The model under review builds one solid part; all positions refer to its coordinate system, in mm. Face numbers are marked on the shaded views. A direction names the side the tool comes from. Give positions to 0.01 mm unless a question says otherwise; leave off trailing zeros. Order: outer loops, then holes, each group sorted by start corner. A loop starts at its lowest first (then second) coordinate and runs counter-clockwise, first axis right, second up. Notation, with made-up numbers: (87.25, -36.5) - (94.25, -36.5) arc R19 ccw to (94.25, 0.5) - close; hole circle Ø8 at (-25, 4.5). An arc over 180 degrees is marked (long way). Answer as CSV lines item,"result". Start each with the question number.
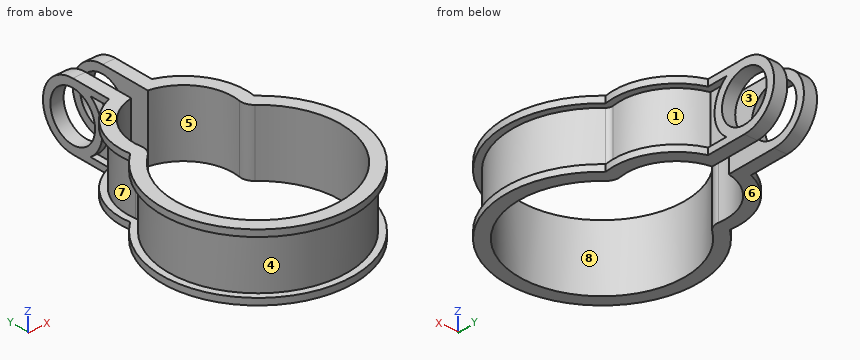
Autodesk Inventor part; units mm, degrees
ref_plane "Work Plane1" through (-2.5, 39.7902, 10) normal (1, 0, 0) x (0, 1, 0)
ref_plane "XZ Plane" through (0, 0, 0) normal (0, 1, 0) x (-1, 0, 0)
ref_plane "XY Plane" through (0, 0, 0) normal (0, 0, 1) x (1, 0, 0)
sketch "Sketch1" plane through (0, 0, 0) normal (0, 0, 1) x (1, 0, 0)
  arc A0 (-16.1874, 19.0517) -> (16.1874, 19.0517) centre (0, 0) ccw
  line L0 (-2.5, 50.7018) -> (-2.5, 39.7902) construction
  line L1 (2.5, 50.7018) -> (2.5, 39.7902) construction
  line L2 (2.5, 50.7018) -> (-2.5, 50.7018) construction
  arc A1 (14.8242, 22.7105) -> (2.5, 39.7902) centre (0, 25) ccw
  arc A2 (-2.5, 39.7902) -> (-14.8242, 22.7105) centre (0, 25) ccw
  arc A3 (-16.1874, 19.0517) -> (-14.8242, 22.7105) centre (-18.7774, 22.1) ccw
  arc A4 (14.8242, 22.7105) -> (16.1874, 19.0517) centre (18.7774, 22.1) ccw
  dimension "d0" = 25
  dimension "d2" = 25
  dimension "d3" = 5
  dimension "d4" = 4
sketch "Sketch2" plane through (0, 0, 0) normal (1, 0, 0) x (0, 1, 0)
  line L0 (-25, 10) -> (-25, -10)
  line L1 (-25, -10) -> (-29, -10)
  line L2 (-29, -10) -> (-29, -8)
  line L3 (-29, -8) -> (-27, -8)
  line L4 (-27, -8) -> (-27, 8)
  line L5 (-27, 8) -> (-29, 8)
  line L6 (-29, 8) -> (-29, 10)
  line L7 (-29, 10) -> (-25, 10)
  line L8 (19.0517, 0) -> (-25, 0)
  point P0 (0, 0)
  point P1 (19.0517, 0)
  dimension "d5" = 20
  dimension "d6" = 2
  dimension "d8" = 4
  dimension "d9" = 2
sweep "Sweep1" add profiles "Sketch2" path "Sketch1"
ref_plane "Work Plane1" through (-2.5, 39.7902, 10) normal (1, 0, 0) x (0, 1, 0)
sketch "Sketch3" plane through (-2.5, 39.7902, 10) normal (1, 0, 0) x (0, 1, 0)
  line L0 (0, 0) -> (0, -20)
  line L1 (0, -20) -> (15.2098, -20)
  arc A0 (15.2098, -20) -> (15.2098, 0) centre (15.2098, -10) ccw
  line L2 (15.2098, 0) -> (0, 0)
  line L3 (3.9441, 0) -> (3.9441, -2)
  point P0 (-39.7902, -10)
  dimension "d12" = 55
extrude "Extrusion1" add sketch "Sketch3" against normal blind 2
sketch "Sketch4" plane through (-4.5, 39.7902, 10) normal (-1, 0, 0) x (0, 0, 1)
  line L0 (-2, 3.6692) -> (-2, 1.6034) construction
  line L1 (0, 3.6692) -> (0, 15.2098)
  arc A0 (0, 15.2098) -> (-20, 15.2098) centre (-10, 15.2098) ccw
  line L2 (-20, 15.2098) -> (-20, 3.6692)
  arc A1 (-18, 9.2098) -> (-2, 9.2098) centre (-10, 15.2098) ccw
  line L3 (-20, 3.6692) -> (-20, 1.6034)
  line L4 (-20, 3.9441) -> (-20, 0)
  line L5 (-18, 1.6034) -> (-18, 9.2098)
  line L6 (-18, 1.972) -> (-18, 3.9441)
  line L7 (-18, 1.6034) -> (-20, 1.6034)
  line L8 (0, 3.6692) -> (0, 1.6034)
  line L9 (0, -17.6902) -> (0, 3.9441)
  line L10 (0, 1.6034) -> (-2, 1.6034)
  line L11 (-2, 1.6034) -> (-2, 9.2098)
  point P0 (-10, -39.7902)
extrude "Extrusion2" add sketch "Sketch4" along normal blind 2
mirror "Mirror1" about plane through (0, 0, 0) normal (1, 0, 0) of "Extrusion1", "Extrusion2"
sketch "Sketch5" plane through (-6.5, 39.7902, 10) normal (-1, 0, 0) x (0, 0, 1)
  arc A0 (0, 15.2098) -> (-20, 15.2098) centre (-10, 15.2098) ccw
  point P0 (-10, -39.7902)
hole "Hole1" at (-6.5, 55, 0) direction (1, 0, 0) diameter 15 end through all
properties part number "Part015. Double clip" material "Steel, Carbon"
Item 1: Take a section at A-A on y = 0. Write out the cut boundary in (x, z), and give its area (3 significant figures).
Item 2: For line 1 along X through (y, z) = (0, 3.75); line 2 along Z through (x, y) = (5, 55); line 3 along X through (y, z) = (25, 3.75), list the stretches that pass through material, from the lowest coordinate up.
Item 3: Take a section at C-C on x = 0. Write out the cut boundary in (y, z).
Item 4: Take a section at D-D on x = -21. Write out the cut boundary in (y, z).
Item 5: Clearance check with flat-ended pins moving along their axes: pin 1 (1.5 mm diameter, centred on y = 30, z = -2.5, fed in from -X); pin 2 (1 mm diameter, centred on x = -11, z = 0.5, fed in from -Y); pin 3 (2 mm diameter, centred on y = 37.5, z = -6, fed in from +X); pin 4 (9 mm diameter, centred on y = 55, z = 0, fed in from +X). State where each tip first meets the part, or that it passes through.
Item 6: Mouldability with a two-part tool opening along Z and no side actions: class the marked faces 6, 7 and 8 as released by +Z, released by -Z, zero draft, split by the parting line, or undercut.
Item 7: Machinability: for the marked faces 1, 2, 3, 4 and 5, which of the approach directions +Z, -Z, +X, -X, +Y, -Y give a long, thin tool a straight path to every point of the face, cutting with its end or side? Answer none if there is none.
Item 8: Take a section at B-B on z = 2. Count the separate pieces of the cut face and the enclosed holes in it, and give its area (3 significant figures).
Data:
1,outline,"(-29, -10) - (-25, -10) - (-25, 10) - (-29, 10) - (-29, 8) - (-27, 8) - (-27, -8) - (-29, -8) - close; (25, -10) - (29, -10) - (29, -8) - (27, -8) - (27, 8) - (29, 8) - (29, 10) - (25, 10) - close"
1,area,"96.0 mm^2"
2,line 1,"x = -27 to -25, 25 to 27"
2,line 2,"z = -10 to -7.5, 7.5 to 10"
2,line 3,"x = -17 to -15, 15 to 17"
3,outline,"(-29, -10) - (-25, -10) - (-25, 10) - (-29, 10) - (-29, 8) - (-27, 8) - (-27, -8) - (-29, -8) - close"
4,outline,"(-20, -10) - (-13.56, -10) - (-13.56, 10) - (-20, 10) - (-20, 8) - (-16.97, 8) - (-16.97, -8) - (-20, -8) - close; (13.56, -10) - (20, -10) - (20, -8) - (16.97, -8) - (16.97, 8) - (20, 8) - (20, 10) - (13.56, 10) - close"
5,pin 1,"stops at x = -16.46"
5,pin 2,"stops at y = -24.87"
5,pin 3,"stops at x = 12.52"
5,pin 4,"passes through"
6,face 6,"released by -Z"
6,face 7,"undercut"
6,face 8,"zero draft"
7,face 1,"+X"
7,face 2,"+Z, +X, -X, +Y, -Y"
7,face 3,"+Z, -Z, +Y"
7,face 4,"none"
7,face 5,"+Z, -Z"
8,separate pieces,"3"
8,enclosed holes,"0"
8,area,"421 mm^2"
